Input: part model. Units: mm. Frame: model coordinates. A direction names the side the tool comes from. Give positions to 0.01 mm unless a question says otherwise; leave off trailing zeros. Loops run counter-clockwise (first coordinate to the right, second up) from the corner with the lowest first, then second, coordinate; pieces in that order, holes last. Notation, with made-up numbers: (-37.75, -28.75) - (-29.75, -28.75) arc R35 cw to (-29.75, 7.25) - close; hole circle Ø10 at (73, 43.25). An arc over 180 degrees is marked (long way). One line per item, written item: value.
from build123d import *
from build123d.topology import SkipClean

# Parameters (mm, degrees)
SKETCH1_R                                       = 28.5
SKETCH1_R_2                                     = 19.5
BOSS_EXTRUDE1_DEPTH                             = 2
SKETCH2_R                                       = 1.5
CUT_EXTRUDE1_DEPTH                              = 41.354677548
CIRPATTERN1_COUNT                               = 3
BOSS_EXTRUDE2_START                             = 4.5
SKETCH3_R                                       = 27.5
SKETCH3_R_2                                     = 19.5
BOSS_EXTRUDE2_DEPTH                             = 4.5
SKETCH4_R                                       = 4.5
SKETCH4_R_2                                     = 2.5
BOSS_EXTRUDE3_DEPTH                             = 1
SKETCH5_R                                       = 4
SKETCH5_R_2                                     = 2.5
BOSS_EXTRUDE4_DEPTH                             = 3.5
CIRPATTERN6_COUNT                               = 3
SKETCH8_R                                       = 1.5
CUT_EXTRUDE4_DEPTH                              = 41.825849654
CIRPATTERN7_COUNT                               = 3
SKETCH9_R                                       = 1.5
CUT_EXTRUDE5_DEPTH                              = 42.779181419
CIRPATTERN8_COUNT                               = 6
CUT_EXTRUDE6_START                              = -3.5
SKETCH10_R                                      = 2.5
CUT_EXTRUDE6_DEPTH                              = 3.5
CIRPATTERN9_COUNT                               = 3
SKETCH11_R                                      = 19.5
SKETCH11_R_2                                    = 16.5
BOSS_EXTRUDE5_DEPTH                             = 6.5
SKETCH12_R                                      = 1.6
CUT_EXTRUDE7_DEPTH                              = 10
CIRPATTERN10_COUNT                              = 3
CSK_FOR_M3_FLAT_HEAD_MACHINE_SCREW1_D           = 3.4
CSK_FOR_M3_FLAT_HEAD_MACHINE_SCREW1_CSINK_D     = 6.3
CSK_FOR_M3_FLAT_HEAD_MACHINE_SCREW1_CSINK_ANGLE = 90


with BuildPart() as part:
    # Sketch1 → Boss-Extrude1 (new body)
    with BuildSketch(Plane.XY):
        Circle(SKETCH1_R)
        Circle(SKETCH1_R_2, mode=Mode.SUBTRACT)
    extrude(amount=BOSS_EXTRUDE1_DEPTH)

    # Sketch2 → Cut-Extrude1 (cut, through all)
    with BuildSketch(Plane.XY.offset(2)):
        with Locations((0, 24)):
            Circle(SKETCH2_R)
    cut_extrude1 = extrude(amount=-CUT_EXTRUDE1_DEPTH, mode=Mode.SUBTRACT)

    # CirPattern1: Cut-Extrude1 ×3 about axis
    cirpattern1_axis = Axis((0, 0, 0), (0, 0, 1))
    for i in range(1, CIRPATTERN1_COUNT):
        add(cut_extrude1.rotate(cirpattern1_axis, i * 360 / CIRPATTERN1_COUNT), mode=Mode.SUBTRACT)

    # Sketch3 → Boss-Extrude2 (add)
    with SkipClean():  # the faces are left unmerged after this step: merging them gives an invalid solid
        with BuildSketch(Plane(origin=(0, 0, 0), x_dir=(-1, 0, 0), z_dir=(0, 0, -1)).offset(BOSS_EXTRUDE2_START)):
            Circle(SKETCH3_R)
            Circle(SKETCH3_R_2, mode=Mode.SUBTRACT)
        extrude(amount=-BOSS_EXTRUDE2_DEPTH)

    # Sketch4 → Boss-Extrude3 (add)
    with SkipClean():  # the faces are left unmerged after this step: merging them gives an invalid solid
        with BuildSketch(Plane.XY.offset(2)):
            with Locations(Location((0, 24, 0), (0, 0, 269.999655686))):
                Circle(SKETCH4_R)
            with Locations((0, 24)):
                Circle(SKETCH4_R_2, mode=Mode.SUBTRACT)
        boss_extrude3 = extrude(amount=BOSS_EXTRUDE3_DEPTH)

    # Sketch5 → Boss-Extrude4 (add)
    with SkipClean():  # the faces are left unmerged after this step: merging them gives an invalid solid
        with BuildSketch(Plane.XY.offset(3)):
            with Locations((0, 24)):
                Circle(SKETCH5_R)
            with Locations((0, 24)):
                Circle(SKETCH5_R_2, mode=Mode.SUBTRACT)
        boss_extrude4 = extrude(amount=BOSS_EXTRUDE4_DEPTH)

    # CirPattern6: Boss-Extrude3, Boss-Extrude4 ×3 about axis
    with SkipClean():  # the faces are left unmerged after this step: merging them gives an invalid solid
        cirpattern6_axis = Axis((0, 0, 0), (0, 0, 1))
        add([boss_extrude3.rotate(cirpattern6_axis, i * 360 / CIRPATTERN6_COUNT) for i in range(1, CIRPATTERN6_COUNT)])
        add([boss_extrude4.rotate(cirpattern6_axis, i * 360 / CIRPATTERN6_COUNT) for i in range(1, CIRPATTERN6_COUNT)])

    # Sketch8 → Cut-Extrude4 (cut, through all)
    with SkipClean():  # the faces are left unmerged after this step: merging them gives an invalid solid
        with BuildSketch(Plane.XY):
            with Locations((0, 24)):
                Circle(SKETCH8_R)
        cut_extrude4 = extrude(amount=-CUT_EXTRUDE4_DEPTH, mode=Mode.SUBTRACT)

    # CirPattern7: Cut-Extrude4 ×3 about axis
    with SkipClean():  # the faces are left unmerged after this step: merging them gives an invalid solid
        cirpattern7_axis = Axis((0, 0, 0), (0, 0, 1))
        for i in range(1, CIRPATTERN7_COUNT):
            add(cut_extrude4.rotate(cirpattern7_axis, i * 360 / CIRPATTERN7_COUNT), mode=Mode.SUBTRACT)

    # Sketch9 → Cut-Extrude5 (cut, through all)
    with SkipClean():  # the faces are left unmerged after this step: merging them gives an invalid solid
        with BuildSketch(Plane(origin=(0, 0, -4.5), x_dir=(-1, 0, 0), z_dir=(0, 0, -1))):
            with Locations((-20.784609691, 12)):
                Circle(SKETCH9_R)
        cut_extrude5 = extrude(amount=-CUT_EXTRUDE5_DEPTH, mode=Mode.SUBTRACT)

    # CirPattern8: Cut-Extrude5 ×6 about axis, 3 skipped
    with SkipClean():  # the faces are left unmerged after this step: merging them gives an invalid solid
        cirpattern8_axis = Axis((0, 0, -4.5), (0, 0, -1))
        add([cut_extrude5.rotate(cirpattern8_axis, i * 360 / CIRPATTERN8_COUNT) for i in range(1, CIRPATTERN8_COUNT) if i not in (1, 3, 5)], mode=Mode.SUBTRACT)

    # Sketch10 → Cut-Extrude6 (cut)
    with SkipClean():  # the faces are left unmerged after this step: merging them gives an invalid solid
        with BuildSketch(Plane.XY.offset(2).offset(CUT_EXTRUDE6_START)):
            with Locations((0, 24)):
                Circle(SKETCH10_R)
        cut_extrude6 = extrude(amount=CUT_EXTRUDE6_DEPTH, mode=Mode.SUBTRACT)

    # CirPattern9: Cut-Extrude6 ×3 about axis
    with SkipClean():  # the faces are left unmerged after this step: merging them gives an invalid solid
        cirpattern9_axis = Axis((0, 0, 0), (0, 0, -1))
        for i in range(1, CIRPATTERN9_COUNT):
            add(cut_extrude6.rotate(cirpattern9_axis, i * 360 / CIRPATTERN9_COUNT), mode=Mode.SUBTRACT)

    # Sketch11 → Boss-Extrude5 (add)
    with SkipClean():  # the faces are left unmerged after this step: merging them gives an invalid solid
        with BuildSketch(Plane(origin=(0, 0, -4.5), x_dir=(-1, 0, 0), z_dir=(0, 0, -1))):
            Circle(SKETCH11_R)
            Circle(SKETCH11_R_2, mode=Mode.SUBTRACT)
        extrude(amount=-BOSS_EXTRUDE5_DEPTH)

    # Sketch12 → Cut-Extrude7 (cut)
    with SkipClean():  # the faces are left unmerged after this step: merging them gives an invalid solid
        with BuildSketch(Plane(origin=(0, 0, -4.5), x_dir=(-1, 0, 0), z_dir=(0, 0, -1))):
            with Locations((10, 17.320508076)):
                Circle(SKETCH12_R)
        cut_extrude7 = extrude(amount=-CUT_EXTRUDE7_DEPTH, mode=Mode.SUBTRACT)

    # CirPattern10: Cut-Extrude7 ×3 about axis
    with SkipClean():  # the faces are left unmerged after this step: merging them gives an invalid solid
        cirpattern10_axis = Axis((0, 0, 0), (0, 0, 1))
        for i in range(1, CIRPATTERN10_COUNT):
            add(cut_extrude7.rotate(cirpattern10_axis, i * 360 / CIRPATTERN10_COUNT), mode=Mode.SUBTRACT)

    # CSK for M3 Flat Head Machine Screw1 (through all)
    with Locations(Plane(origin=(-20.784609691, 12, 2), x_dir=(1, 0, 0), z_dir=(0, 0, 1))):
        with Locations((0, 0), (41.569219382, 0), (20.784609691, -36)):
            CounterSinkHole(CSK_FOR_M3_FLAT_HEAD_MACHINE_SCREW1_D / 2, CSK_FOR_M3_FLAT_HEAD_MACHINE_SCREW1_CSINK_D / 2, counter_sink_angle=CSK_FOR_M3_FLAT_HEAD_MACHINE_SCREW1_CSINK_ANGLE)


solid = part.part
Item 1: Section A-A, the plane y = 0. Output: boundary loops of the cut face in (x, z).
Verdict:
outline: (-28.5, 0) - (-27.5, 0) - (-27.5, -4.5) - (-16.5, -4.5) - (-16.5, 2) - (-28.5, 2) - close; (16.5, -4.5) - (18.4, -4.5) - (18.4, 2) - (16.5, 2) - close; (21.6, -4.5) - (27.5, -4.5) - (27.5, 0) - (28.5, 0) - (28.5, 2) - (21.6, 2) - close
Item 2: Material intervals for L1, parallel to Y at x = 0, z = -0.25; L2, parallel to X at y = -12, z = 1.25; L3, parallel to X at y = 12, z = -1.05, sorted ascending.
Verdict:
L1: y = -27.5 to -25.7, -22.3 to -16.5, 16.5 to 21.5, 26.5 to 27.5
L2: x = -25.85 to -23.28, -18.28 to -11.32, 11.32 to 18.28, 23.28 to 25.85
L3: x = -24.74 to -22.48, -19.08 to -11.32, 11.32 to 19.08, 22.48 to 24.74
Item 3: Access query for faces 1 (the face through (-18, -13, 6.5)), 2 (the face through (-2.7, 27.6, 2.5)). Directions: +Z, -Z, +X, -X, +Y, -Y. A direction counts if a zero-diameter tool reaches every point of the face in a straight line with its end or side. Return the directions, or none.
Verdict:
face 1: +Z, +X, -X, +Y, -Y
face 2: +Z
Item 4: Section D-D, the plane z = -3.25. Count the separate pieces of the cut face and the enclosed holes in it, and give its area (3 significant figures).
Verdict:
separate pieces: 1
enclosed holes: 10
area: 1,450 mm^2
Item 5: Pin query (flat end, axial travel): P1, Ø1.5, axis at x = 21.5, y = -11, coming from the +Z side; P2, Ø1, axis at x = 12, z = 0.5, coming from the -Y side; P3, Ø5, axis at x = 12, z = -0.5, coming from the +Y side. Return the tip coordinate at first contact, or that it passes through.
Verdict:
P1: stops at z = -1.5
P2: stops at y = -26.08
P3: stops at y = 26.85
Item 6: Section B-B, the plane x = -10. Output: boundary loops of the cut face in (y, z), and give its area (3 significant figures).
Verdict:
outline: (-26.69, 0) - (-25.62, 0) - (-25.62, -4.5) - (-18.92, -4.5) - (-18.92, 2) - (-26.69, 2) - close; (-15.72, -4.5) - (-13.12, -4.5) - (-13.12, 2) - (-15.72, 2) - close; (13.12, -4.5) - (15.72, -4.5) - (15.72, 2) - (13.12, 2) - close; (18.92, -4.5) - (25.62, -4.5) - (25.62, 0) - (26.69, 0) - (26.69, 2) - (18.92, 2) - close
area: 125 mm^2
Item 7: Draft query along X for faces 3 (the face through (-14.9, 23.4, 0)), 4 (the face through (-20.09, -13.33, -2.98)), 5 (the face through (-16.323, -11.414, 2.493)), 6 (the face through (-0.521, 27.966, 4.726)). Return one class per face: pulls with the +X half, pulls with the -X half, needs draft (parallel to the pull), parting line crosses it, or undercut.
Verdict:
face 3: needs draft
face 4: undercut
face 5: undercut
face 6: parting line crosses it
Item 8: Section C-C, the plane y = 12. Output: boundary loops of the cut face in (x, z), and give its area (3 significant figures).
Verdict:
outline: (-25.85, 0) - (-24.74, 0) - (-24.74, -4.5) - (-22.48, -4.5) - (-22.48, 0.55) - (-23.93, 2) - (-25.85, 2) - close; (-19.08, -4.5) - (-11.32, -4.5) - (-11.32, 2) - (-17.63, 2) - (-19.08, 0.55) - close; (11.32, -4.5) - (19.08, -4.5) - (19.08, 0.55) - (17.63, 2) - (11.32, 2) - close; (22.48, -4.5) - (24.74, -4.5) - (24.74, 0) - (25.85, 0) - (25.85, 2) - (23.93, 2) - (22.48, 0.55) - close
area: 130 mm^2
